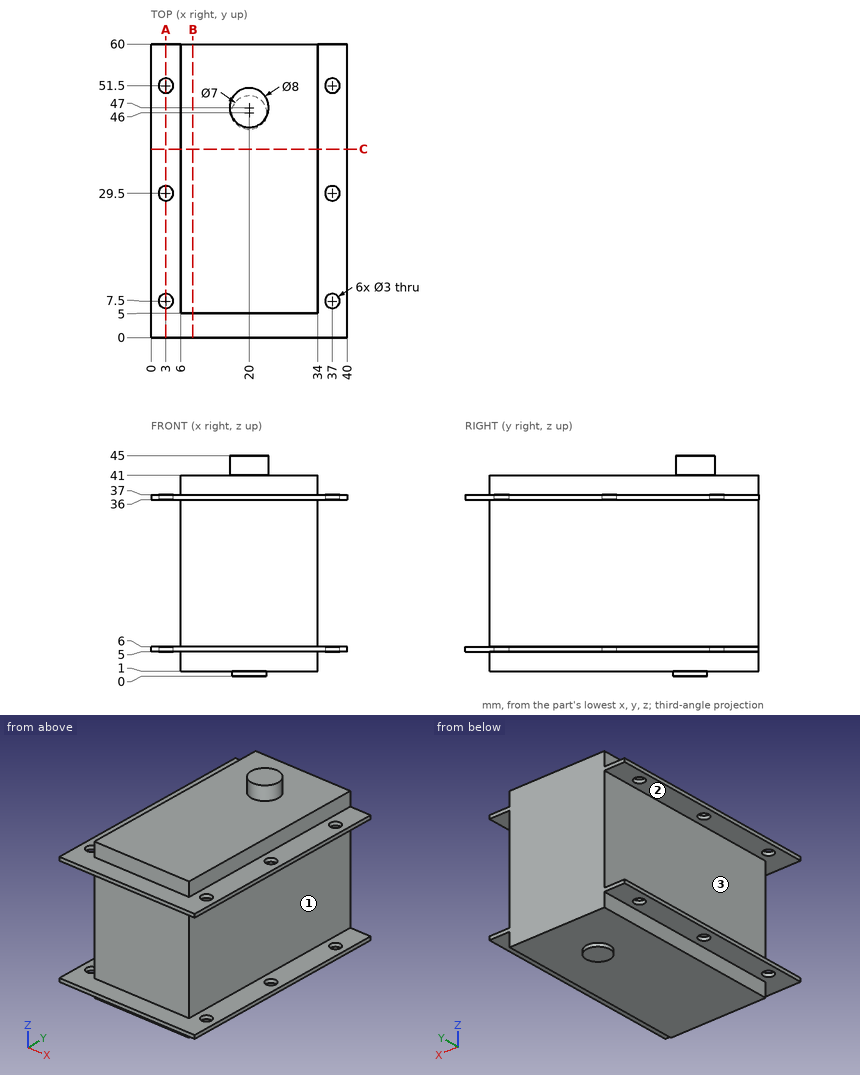
Study the drawing (mm; zero at the part's minimum x, y, z) and answer. A direction names the side the tool comes from. Coordinates: 2 decimals unless noted, no trailing zeros. Loops run counter-clockwise (first coordinate to the right, second up) from the corner with the lowest first, then second, coordinate; pieces in that order, holes last. Notation, with made-up numbers: M 26,84.5 L 40,84.5 A15 ccw 40,89.5 Z; hole C -17.5,-34.75 d9. An arc over 180 degrees is marked long. Answer in a Markdown table with one row per item. Add a question column.
1. A tool of negligible diameter and unlimited length cuts with its end or side. For the marked faces 1, 2 and 3, from which of +Z, -Z, +X, -X, +Y, -Y can it reach the whole face along a straight path? Write none if from no direction.
2. Consider L1, parallel to X at y = 29.5, z = 36.35; L2, parallel to Z at x = 3, y = 42; L3, parallel to Y at x = 28.5, z = 25. Determine where each line is inside the solid, lowest interval first.
3. Find section B-B, the plane x = 8.5. Write down the section's boundary in (y, z), then the cut area to 3 significant figures.
4. Find section A-A, the plane x = 3. State how many separate pieces and enclosed holes the cut face has, then the cut area to 3 significant figures.
5. Flat-ended cylindrical pins translate along their axes: P1, Ø12, axis at x = 17.5, y = 24, coming from the -Z side; P2, Ø4, axis at x = 3, y = 51.5, coming from the +Z side; P3, Ø8.5, axis at x = 26, z = 15, coming from the -Y side; P4, Ø1.8, axis at x = 37, y = 29.5, coming from the +Z side. Find the tip coordinate at first contact, or state that the pin passes through.
6. Find section C-C, the plane y = 38.5. Write down the section's boundary in (x, z).
Reported:
| question | item | result |
|---|---|---|
| 1 | face 1 | +X, +Y, -Y |
| 1 | face 2 | -Y |
| 1 | face 3 | -X, +Y, -Y |
| 2 | L1 | x = 0 to 1.5, 4.5 to 35.5, 38.5 to 40 |
| 2 | L2 | z = 5 to 6, 36 to 37 |
| 2 | L3 | y = 5 to 60 |
| 3 | outline | M 0,5 L 5,5 L 5,1 L 60,1 L 60,41 L 5,41 L 5,37 L 0,37 L 0,36 L 5,36 L 5,6 L 0,6 Z |
| 3 | area | 2,210 mm^2 |
| 4 | separate pieces | 8 |
| 4 | enclosed holes | 0 |
| 4 | area | 102 mm^2 |
| 5 | P1 | stops at z = 1 |
| 5 | P2 | stops at z = 37 |
| 5 | P3 | stops at y = 5 |
| 5 | P4 | passes through |
| 6 | outline | M 0,5 L 6,5 L 6,1 L 34,1 L 34,5 L 40,5 L 40,6 L 34,6 L 34,36 L 40,36 L 40,37 L 34,37 L 34,41 L 6,41 L 6,37 L 0,37 L 0,36 L 6,36 L 6,6 L 0,6 Z |
